For this review, use the dimensioned drawing (mm, ordinates from the lowest corner) and the shaded views. Round coordinates to 2 decimals unless told otherwise and drop trailing zeros. Write each loop counter-clockwise with the first axis right and the second up, starting at its lowest first coordinate (ties: lowest second). Pieces come first, ordered by that corner, then holes. Notation, with made-up numbers: (19.5, -25.5) -> (28.5, -25.5) arc R33 ccw to (28.5, 10.5) -> close; hole circle Ø2 at (77.25, 5.5). An arc over 180 degrees is marked (long way). Answer in a Markdown table with one row per item. Add a question column.
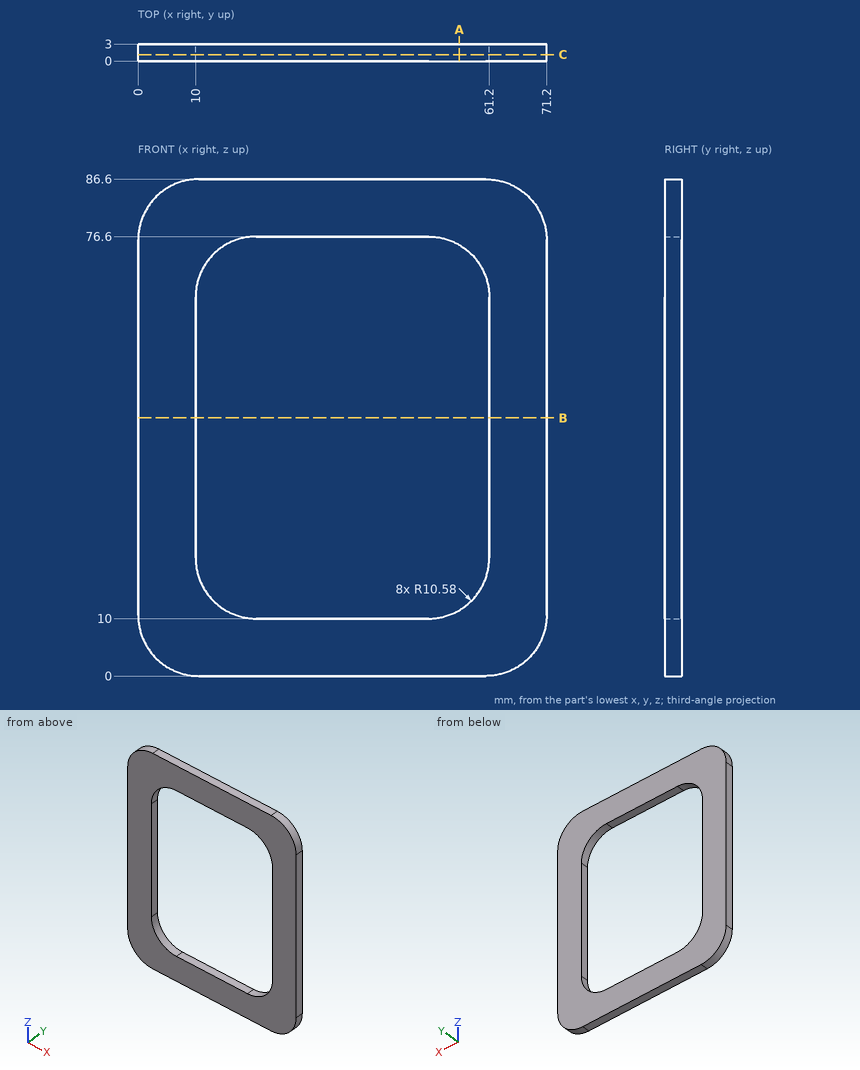
1. For L1, parallel to X at y = 0.7, z = 32; L2, parallel to Z at x = 30, y = 2.45; L3, parallel to Z at x = 55, y = 2, list the stretches that pass through material, from the lowest coordinate up. Write a range as [from, to].
2. We need section A-A (x = 56). Write out the cut boundary in (y, z), plus the area to 3 significant figures.
3. We need section B-B (z = 45). Write out the cut boundary in (x, y), plus the area to 3 significant figures.
4. We need section C-C (y = 1.15). Write out the cut boundary in (x, z), plus the area to 3 significant figures.
Response:
| question | item | result |
|---|---|---|
| 1 | L1 | [0, 10], [61.2, 71.2] |
| 1 | L2 | [0, 10], [76.6, 86.6] |
| 1 | L3 | [0, 10.95], [75.65, 86.6] |
| 2 | outline | (0, 0) -> (3, 0) -> (3, 11.47) -> (0, 11.47) -> close; (0, 75.13) -> (3, 75.13) -> (3, 86.6) -> (0, 86.6) -> close |
| 2 | area | 68.8 mm2 |
| 3 | outline | (0, 0) -> (10, 0) -> (10, 3) -> (0, 3) -> close; (61.2, 0) -> (71.2, 0) -> (71.2, 3) -> (61.2, 3) -> close |
| 3 | area | 60.0 mm2 |
| 4 | outline | (0, 10.58) arc R10.58 ccw to (10.58, 0) -> (60.62, 0) arc R10.58 ccw to (71.2, 10.58) -> (71.2, 76.02) arc R10.58 ccw to (60.62, 86.6) -> (10.58, 86.6) arc R10.58 ccw to (0, 76.02) -> close; hole (10, 20.58) arc R10.58 ccw to (20.58, 10) -> (50.62, 10) arc R10.58 ccw to (61.2, 20.58) -> (61.2, 66.02) arc R10.58 ccw to (50.62, 76.6) -> (20.58, 76.6) arc R10.58 ccw to (10, 66.02) -> close |
| 4 | area | 2,760 mm2 |
